```python
from build123d import *

# Parameters (mm, degrees)
EXTRUDE_1_DEPTH              = 16
SKETCH_3_R                   = 7.5
EXTRUDE_2_DEPTH              = 22
SKETCH_4_R                   = 38.5
CUT_EXTRUDE_1_DEPTH          = 12
CUT_EXTRUDE_2_DEPTH          = 16
CUT_EXTRUDE_3_REACH          = 164.951
CUT_EXTRUDE_3_END_RADIUS     = 18
SKETCH_6_R                   = 2.5
SKETCH_7_R                   = 4.5
CUT_EXTRUDE_4_DEPTH          = 28
HOLE_WIZARD_M8_1_D           = 6.8
HOLE_WIZARD_M8_1_CSINK_D     = 8.05
HOLE_WIZARD_M8_1_CSINK_ANGLE = 90


with BuildPart() as part:
    # 草图1 → 凸台-拉伸1 (new body)
    with BuildSketch(Plane(origin=(0, 0, 0), x_dir=(0, 0, -1), z_dir=(1, 0, 0))):
        with BuildLine():
            Line((-132, 0), (-36, 0))
            ThreePointArc((-36, 0), (-1.000386324, 35.986097693), (35.944401511, 2))
            Line((35.944401511, 2), (56, 2))
            Line((56, 2), (56, 30))
            Line((56, 30), (31.638584039, 30))
            ThreePointArc((31.638584039, 30), (28.354636152, 30.554594436), (25.43494011, 32.156862745))
            ThreePointArc((25.43494011, 32.156862745), (9.982578161, 39.766168199), (-7.231593148, 40.357205807))
            Line((-7.231593148, 40.357205807), (-132, 18))
            Line((-132, 18), (-132, 0))
        make_face()
        with BuildLine():
            ThreePointArc((35.944401511, -2), (-1.000386324, -35.986097693), (-36, 0))
            Line((-36, 0), (-132, 0))
            Line((-132, 0), (-132, -18))
            Line((-132, -18), (-7.231593148, -40.357205807))
            ThreePointArc((-7.231593148, -40.357205807), (9.982578161, -39.766168199), (25.43494011, -32.156862745))
            ThreePointArc((25.43494011, -32.156862745), (28.354636152, -30.554594436), (31.638584039, -30))
            Line((31.638584039, -30), (56, -30))
            Line((56, -30), (56, -2))
            Line((56, -2), (35.944401511, -2))
        make_face()
    extrude(amount=EXTRUDE_1_DEPTH)

    # 草图3 → 凸台-拉伸2 (add)
    with BuildSketch(Plane.XY.offset(132)):
        with BuildLine():
            Line((16, 18), (0, 18))
            Line((0, 18), (0, -18))
            Line((0, -18), (16, -18))
            ThreePointArc((16, -18), (34, 0), (16, 18))
        make_face()
        with Locations(Location((16, 0, 0), (0, 0, 90))):
            Circle(SKETCH_3_R, mode=Mode.SUBTRACT)
    extrude(amount=EXTRUDE_2_DEPTH)

    # 草图4 → 切除-拉伸1 (cut)
    with BuildSketch(Plane.ZY):
        Circle(SKETCH_4_R)
    extrude(amount=-CUT_EXTRUDE_1_DEPTH, mode=Mode.SUBTRACT)

    # 草图5 → 切除-拉伸2 (cut)
    with BuildSketch(Plane(origin=(16, 0, 0), x_dir=(0, 0, -1), z_dir=(1, 0, 0))):
        with BuildLine():
            Line((-132, -9.872579049), (-132, 9.872579049))
            Line((-132, 9.872579049), (-42.206623977, 25.962621701))
            ThreePointArc((-42.206623977, 25.962621701), (-37.309997522, 24.021277058), (-36.869036306, 18.772341655))
            ThreePointArc((-36.869036306, 18.772341655), (-41.373018374, 0), (-36.869036306, -18.772341655))
            ThreePointArc((-36.869036306, -18.772341655), (-37.309997522, -24.021277058), (-42.206623977, -25.962621701))
            Line((-42.206623977, -25.962621701), (-132, -9.872579049))
        make_face()
    extrude(amount=-CUT_EXTRUDE_2_DEPTH, mode=Mode.SUBTRACT)

    # 切除-拉伸3: up to this cylinder (the profile starts inside it)
    cut_extrude_3_end = Plane(origin=(16, 0, 143), z_dir=(0, 0, -1)) * Cylinder(CUT_EXTRUDE_3_END_RADIUS, 366.902, mode=Mode.PRIVATE)
    # 草图6 → 切除-拉伸3 (cut, up to the surface)
    with BuildSketch(Plane.ZY, mode=Mode.PRIVATE) as cut_extrude_3_sk1:
        with Locations((143, 0)):
            Circle(SKETCH_6_R)
    cut_extrude_3_tool1 = extrude(cut_extrude_3_sk1.sketch, amount=-CUT_EXTRUDE_3_REACH, mode=Mode.PRIVATE) & cut_extrude_3_end
    add(cut_extrude_3_tool1.solids().sort_by_distance((0, 0, 143))[0], mode=Mode.SUBTRACT)

    # 草图7 → 切除-拉伸4 (cut)
    with BuildSketch(Plane.XZ.offset(30)):
        with Locations(Location((8, -46, 0), (0, 0, 270))):
            Circle(SKETCH_7_R)
    extrude(amount=-CUT_EXTRUDE_4_DEPTH, mode=Mode.SUBTRACT)

    # M8 螺纹孔1 (through all)
    with Locations(Plane(origin=(0, 30, 0), x_dir=(1, 0, 0), z_dir=(0, 1, 0))):
        with Locations((8, 46)):
            CounterSinkHole(HOLE_WIZARD_M8_1_D / 2, HOLE_WIZARD_M8_1_CSINK_D / 2, counter_sink_angle=HOLE_WIZARD_M8_1_CSINK_ANGLE)


solid = part.part
```
Part model, mm, in its own coordinate system. A direction names the side the tool comes from. Round coordinates to 2 decimals unless told otherwise and drop trailing zeros. Write each loop counter-clockwise with the first axis right and the second up, starting at its lowest first coordinate (ties: lowest second). Pieces come first, ordered by that corner, then holes. Notation, with made-up numbers: (75.25, -16.5) -> (103.25, -16.5) arc R18 cw to (103.25, 2.5) -> close; hole circle Ø3 at (4, 34). An arc over 180 degrees is marked (long way). Return JSON: item names as keys, results as strings. Group by question number.
Q1. Saw through at D-D on x = 31.5. Write the cut outline in (y, z).
Q2. Which spindle directions (+Z, -Z, +X, -X, +Y, -Y) get a long thin tool onto all of the face, cutting with end or side? Do faces 4 (the flat face through (12, 34.4, 11.2)), 5 (the flat face through (8, -18, 143)), 6 (the flat face through (16, 3, 38)). Say none if no direction does.
Q3. Mould opens along Y. For faces 1 (the flat face through (8, -2, -51)), 2 (the flat face through (0, 0, 41)), 3 (the cylindrical face through (34, 0, 140)) say: pulls with the +Y half, pulls with the -Y half, needs draft (parallel to the pull), parting line crosses it, or undercut.
Q4. Saw through at C-C on y = -15.5. Write the cut outline in (x, z), plus the area to 3 significant figures.
Q5. Saw through at A-A on z = 0. Write the cut outline in (x, y).
Q6. Pin check, flat tips, straight feed: pin 1 (8 mm diameter, centred on x = 8, z = -46, fed in from +Y) (3 decimals); pin 2 (3 mm diameter, centred on x = 15, z = 91, fed in from -Y); pin 3 (8 mm diameter, centred on x = 9.5, z = 145.5, fed in from -Y). Stop position of each tip, or through.
Q7. Probe L1, parallel to Y at x = 4, z = 143; L2, parallel to Z at x = 10, y = -3; L3, parallel to Y at x = 16, z = 140. List the from-to ranges inside material, lowest first. Write a range as [from, to].
Q8. Saw through at B-B on z = -46. Write the cut outline in (x, y) (3 decimals), plus the area to 3 significant figures.
Answer:
{
 "1": {"outline": "(-9.15, 132) -> (9.15, 132) -> (9.15, 154) -> (-9.15, 154) -> close; hole circle Ø5 at (0, 143)"},
 "2": {"face 4": "-X", "face 5": "+Z, +X, -X, -Y", "face 6": "-Z, +X, +Y, -Y"},
 "3": {"face 1": "undercut", "face 2": "needs draft", "face 3": "parting line crosses it"},
 "4": {"outline": "(0, -56) -> (16, -56) -> (16, -32.49) -> (12, -32.49) -> (12, -35.24) -> (0, -35.24) -> close; (0, 35.24) -> (12, 35.24) -> (12, 32.49) -> (16, 32.49) -> (16, 38.36) -> (0, 38.36) -> close; (0, 100.6) -> (16, 100.6) -> (16, 132) -> (25.15, 132) -> (25.15, 154) -> (0, 154) -> close; hole circle Ø9 at (8, -46)", "area": "1,400 mm2"},
 "5": {"outline": "(0, -41) -> (16, -41) -> (16, -36) -> (12, -36) -> (12, -38.5) -> (0, -38.5) -> close; (0, 38.5) -> (12, 38.5) -> (12, 36) -> (16, 36) -> (16, 41) -> (0, 41) -> close"},
 "6": {"pin 1": "y = 29.975", "pin 2": "y = -25.62", "pin 3": "y = -18"},
 "7": {"L1": "[-18, -2.5], [2.5, 18]", "L2": "[-56, -50.03], [-41.97, -38.38], [38.38, 41.26]", "L3": "[-18, -7.5], [7.5, 18]"},
 "8": {"outline": "(0, -30) -> (3.5, -30) -> (3.5, -2) -> (0, -2) -> close; (0, 2) -> (4.6, 2) -> (4.6, 29.375) -> (3.975, 30) -> (0, 30) -> close; (11.4, 2) -> (16, 2) -> (16, 30) -> (12.025, 30) -> (11.4, 29.375) -> close; (12.5, -30) -> (16, -30) -> (16, -2) -> (12.5, -2) -> close", "area": "453 mm2"}
}
